Could you check a few things on this drawing? It's one solid part, dimensions in mm from its lowest x, y, z. Round coordinates to 2 decimals unless told otherwise and drop trailing zeros. Write each loop counter-clockwise with the first axis right and the second up, starting at its lowest first coordinate (ties: lowest second). Pieces come first, ordered by that corner, then holes. Notation, with made-up numbers: (41, -19.5) -> (71, -19.5) arc R9 cw to (71, -14.5) -> close; hole circle Ø2 at (-26.75, 34.25). An arc over 180 degrees is marked (long way). Return JSON: item names as keys, results as strings.
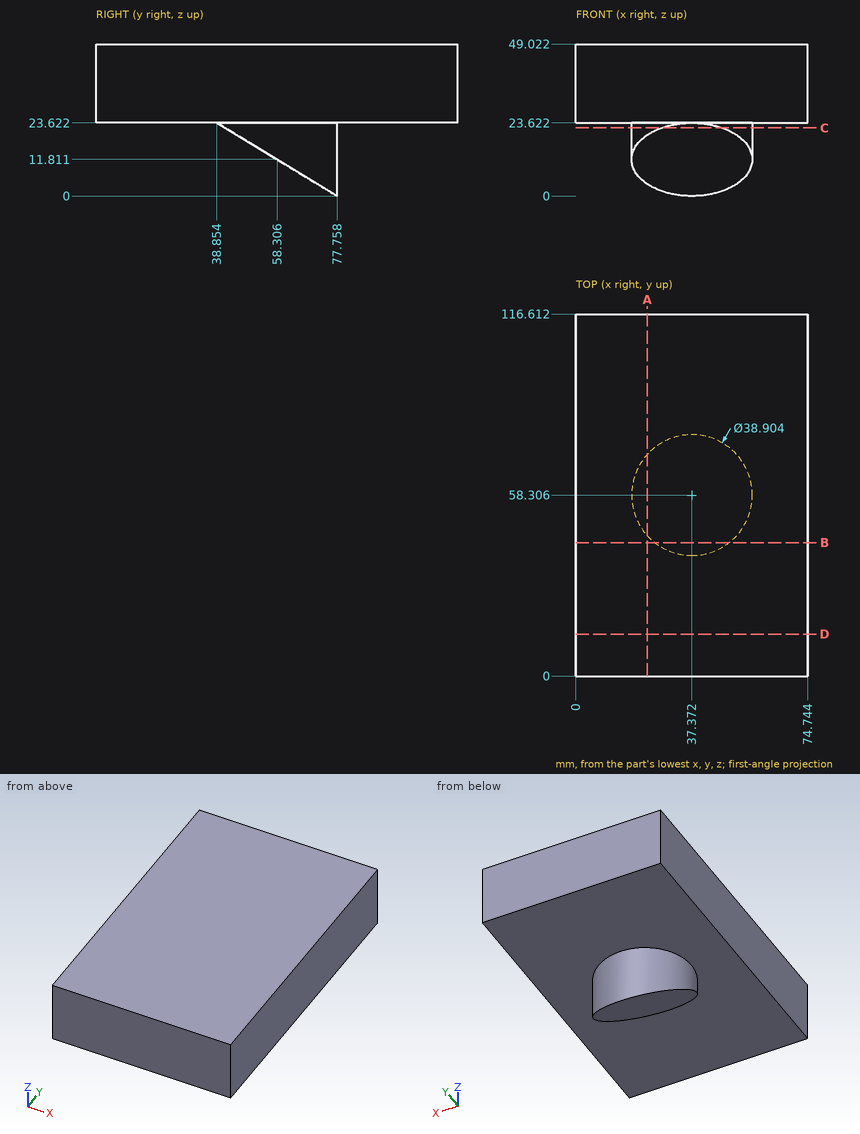
1) I want a section at D-D, the plane y = 13.5. Please give me the cut outline in (x, z) (1 decimal).
Return value:
{"outline": "(0, 23.6) -> (74.7, 23.6) -> (74.7, 49) -> (0, 49) -> close"}
2) If I drill on probe 1 along Z at (x, y) = (24, 106); probe 2 along Z at (x, y) = (42.5, 71) (1 decimal); probe 3 along X at (y, z) = (67.5, 9) (1 decimal), over which ranges is the centre line in solid material (lowest first)? Write a range as [from, to].
Return value:
{"probe 1": "[23.62, 49.02]", "probe 2": "[4.1, 49]", "probe 3": "[20.2, 54.5]"}
3) I want a section at C-C, the plane z = 22. Please give me the cut outline in (x, y) (1 decimal), and give its area (3 significant figures).
Return value:
{"outline": "(27.5, 41.5) -> (47.2, 41.5) arc R19.5 ccw (long way) to start", "area": "1,150 mm²"}
4) Will these pins go through, and if not, where does the flat tip stop? pin 1 Ø10 at (x, z) = (59.5, 14) entering from -Y (1 decimal); pin 2 Ø6 at (x, z) = (56.5, 19.5) entering from +Y; pin 3 Ø6 at (x, y) = (14, 18) entering from -Z.
Return value:
{"pin 1": "y = 50.5", "pin 2": "y = 69.18", "pin 3": "z = 23.62"}
5) I want a section at B-B, the plane y = 43. Please give me the cut outline in (x, z) (1 decimal).
Return value:
{"outline": "(0, 23.6) -> (25.4, 23.6) -> (25.4, 21.1) -> (49.4, 21.1) -> (49.4, 23.6) -> (74.7, 23.6) -> (74.7, 49) -> (0, 49) -> close"}
6) I want a section at A-A, the plane x = 23. Please give me the cut outline in (y, z), and give its area (3 significant figures).
Return value:
{"outline": "(0, 23.62) -> (45.2, 23.62) -> (45.2, 19.77) -> (71.41, 3.85) -> (71.41, 23.62) -> (116.61, 23.62) -> (116.61, 49.02) -> (0, 49.02) -> close", "area": "3,270 mm²"}
